Could you check a few things on this model? Use its own coordinates, in mm. A direction names the side the tool comes from. Give positions to 0.01 mm unless a question says otherwise; leave off trailing zeros. Loops run counter-clockwise (first coordinate to the right, second up) from the corner with the lowest first, then second, coordinate; pieces in that order, holes last. Notation, with made-up numbers: M 45,88 L 65,88 A29 ccw 65,124 Z; hole C 1.5,73.25 d9. An arc over 180 degrees is marked long. Answer in a Markdown table with one row per item. Add a question column.
1. Thinking about a two-plate mould opening in X: for faces 3 (the cylindrical face through (173.486, 211.797, -0.76)), 4 (the flat face through (128, 106, -1.5)), 5 (the cylindrical face through (247.34, 11.55, -0.76)), 6 (the cylindrical face through (4.51, 248.22, -0.76)), which applies, released by +X, released by -X, zero draft, split by the parting line, or undercut?
2. If we section it at A-A on x = 57.5: List the corners of the cut face in (y, z) for me.
3. I need wall thicknesses on line 1 along X through (y, z) = (257.5, -0.4); line 2 along Y through (x, z) = (19.5, -1.1); line 3 along X through (y, z) = (221.5, -1). Which ranges of each line are inside material? Lowest first, please. Write a range as from..to.
4. Which directions (+Z, -Z, +X, -X, +Y, -Y) give clear straight access to the entire face, cutting with the end or side of a thin tool? Please do faces 1 (the cylindrical face through (197.01, 265.15, -0.76)), 2 (the cylindrical face through (85.203, 211.486, -0.76)).
5. If we section it at B-B on z = -1.05: Count the separate pieces of the cut face and the enclosed holes in it, then the cut area to 3 significant figures.
```python
from build123d import *

# Parameters (mm, degrees)
CONVERT_SOLID1_START       = -1.5
CONVERT_SOLID1_OUTLINE_R   = 2.6
CONVERT_SOLID1_OUTLINE_R_2 = 1.65
CONVERT_SOLID1_OUTLINE_R_3 = 3.5
CONVERT_SOLID1_OUTLINE_R_4 = 10
CONVERT_SOLID1_DEPTH       = 1.5


# Read off the part's stored shape, not the designer's step: Convert-Solid1
with BuildPart() as part:
    # Convert-Solid1 outline → Convert-Solid1 (new body)
    with BuildSketch(Plane.XY.offset(CONVERT_SOLID1_START)):
        with BuildLine():
            ThreePointArc((204, 268), (196.928932188, 265.071067812), (194, 258))
            Line((194, 258), (194, 253))
            ThreePointArc((194, 253), (193.853553391, 252.646446609), (193.5, 252.5))
            Line((193.5, 252.5), (15, 252.5))
            ThreePointArc((15, 252.5), (4.393398282, 248.106601718), (0, 237.5))
            Line((0, 237.5), (0, 30.5))
            ThreePointArc((0, 30.5), (4.393398282, 19.893398282), (15, 15.5))
            Line((15, 15.5), (193.5, 15.5))
            ThreePointArc((193.5, 15.5), (193.853553391, 15.353553391), (194, 15))
            Line((194, 15), (194, 10))
            ThreePointArc((194, 10), (196.928932188, 2.928932188), (204, 0))
            Line((204, 0), (249, 0))
            ThreePointArc((249, 0), (256.071067812, 2.928932188), (259, 10))
            Line((259, 10), (259, 258))
            ThreePointArc((259, 258), (256.071067812, 265.071067812), (249, 268))
            Line((249, 268), (204, 268))
        make_face()
        with Locations((10.5, 50)):
            Circle(CONVERT_SOLID1_OUTLINE_R, mode=Mode.SUBTRACT)
        with Locations((19.5, 60.5)):
            Circle(CONVERT_SOLID1_OUTLINE_R, mode=Mode.SUBTRACT)
        with Locations((10.5, 71)):
            Circle(CONVERT_SOLID1_OUTLINE_R, mode=Mode.SUBTRACT)
        with Locations((82.529437252, 120.529437252)):
            Circle(CONVERT_SOLID1_OUTLINE_R_2, mode=Mode.SUBTRACT)
        with Locations((209, 10.5)):
            Circle(CONVERT_SOLID1_OUTLINE_R_3, mode=Mode.SUBTRACT)
        with Locations((218.380820142, 10.5)):
            Circle(CONVERT_SOLID1_OUTLINE_R_2, mode=Mode.SUBTRACT)
        with Locations((233.880820142, 10.5)):
            Circle(CONVERT_SOLID1_OUTLINE_R_2, mode=Mode.SUBTRACT)
        with Locations((244, 10.5)):
            Circle(CONVERT_SOLID1_OUTLINE_R_3, mode=Mode.SUBTRACT)
        with Locations((212.5, 46.5)):
            Circle(CONVERT_SOLID1_OUTLINE_R_2, mode=Mode.SUBTRACT)
        with Locations((226.5, 60.5)):
            Circle(CONVERT_SOLID1_OUTLINE_R_4, mode=Mode.SUBTRACT)
        with Locations((240.5, 46.5)):
            Circle(CONVERT_SOLID1_OUTLINE_R_2, mode=Mode.SUBTRACT)
        with Locations((129.5, 113.5)):
            Circle(CONVERT_SOLID1_OUTLINE_R_2, mode=Mode.SUBTRACT)
        with Locations((176.470562748, 120.529437252)):
            Circle(CONVERT_SOLID1_OUTLINE_R_2, mode=Mode.SUBTRACT)
        with Locations((212.5, 74.5)):
            Circle(CONVERT_SOLID1_OUTLINE_R_2, mode=Mode.SUBTRACT)
        with Locations((240.5, 74.5)):
            Circle(CONVERT_SOLID1_OUTLINE_R_2, mode=Mode.SUBTRACT)
        with Locations((10.5, 197)):
            Circle(CONVERT_SOLID1_OUTLINE_R, mode=Mode.SUBTRACT)
        with Locations((75.5, 167.5)):
            Circle(CONVERT_SOLID1_OUTLINE_R_2, mode=Mode.SUBTRACT)
        with Locations((19.5, 207.5)):
            Circle(CONVERT_SOLID1_OUTLINE_R, mode=Mode.SUBTRACT)
        with Locations((10.5, 218)):
            Circle(CONVERT_SOLID1_OUTLINE_R, mode=Mode.SUBTRACT)
        with Locations((82.529437252, 214.470562748)):
            Circle(CONVERT_SOLID1_OUTLINE_R_2, mode=Mode.SUBTRACT)
        with BuildLine():
            Line((179.5, 197.5), (179.5, 137.5))
            ThreePointArc((179.5, 137.5), (173.642135624, 123.357864376), (159.5, 117.5))
            Line((159.5, 117.5), (99.5, 117.5))
            ThreePointArc((99.5, 117.5), (85.357864376, 123.357864376), (79.5, 137.5))
            Line((79.5, 137.5), (79.5, 197.5))
            ThreePointArc((79.5, 197.5), (85.357864376, 211.642135624), (99.5, 217.5))
            Line((99.5, 217.5), (159.5, 217.5))
            ThreePointArc((159.5, 217.5), (173.642135624, 211.642135624), (179.5, 197.5))
        make_face(mode=Mode.SUBTRACT)
        with Locations((183.5, 167.5)):
            Circle(CONVERT_SOLID1_OUTLINE_R_2, mode=Mode.SUBTRACT)
        with Locations((212.5, 193.5)):
            Circle(CONVERT_SOLID1_OUTLINE_R_2, mode=Mode.SUBTRACT)
        with Locations((240.5, 193.5)):
            Circle(CONVERT_SOLID1_OUTLINE_R_2, mode=Mode.SUBTRACT)
        with Locations((129.5, 221.5)):
            Circle(CONVERT_SOLID1_OUTLINE_R_2, mode=Mode.SUBTRACT)
        with Locations((176.470562748, 214.470562748)):
            Circle(CONVERT_SOLID1_OUTLINE_R_2, mode=Mode.SUBTRACT)
        with Locations((226.5, 207.5)):
            Circle(CONVERT_SOLID1_OUTLINE_R_4, mode=Mode.SUBTRACT)
        with Locations((212.5, 221.5)):
            Circle(CONVERT_SOLID1_OUTLINE_R_2, mode=Mode.SUBTRACT)
        with Locations((240.5, 221.5)):
            Circle(CONVERT_SOLID1_OUTLINE_R_2, mode=Mode.SUBTRACT)
        with Locations((209, 257.5)):
            Circle(CONVERT_SOLID1_OUTLINE_R_3, mode=Mode.SUBTRACT)
        with Locations((218.75, 257.5)):
            Circle(CONVERT_SOLID1_OUTLINE_R_2, mode=Mode.SUBTRACT)
        with Locations((234.25, 257.5)):
            Circle(CONVERT_SOLID1_OUTLINE_R_2, mode=Mode.SUBTRACT)
        with Locations((244, 257.5)):
            Circle(CONVERT_SOLID1_OUTLINE_R_3, mode=Mode.SUBTRACT)
    extrude(amount=CONVERT_SOLID1_DEPTH)


solid = part.part
```
Results:
| question | item | result |
|---|---|---|
| 1 | face 3 | undercut |
| 1 | face 4 | zero draft |
| 1 | face 5 | undercut |
| 1 | face 6 | released by -X |
| 2 | outline | M 15.5,-1.5 L 252.5,-1.5 L 252.5,0 L 15.5,0 Z |
| 3 | line 1 | 194..205.5, 212.5..217.1, 220.4..232.6, 235.9..240.5, 247.5..259 |
| 3 | line 2 | 15.5..57.9, 63.1..204.9, 210.1..252.5 |
| 3 | line 3 | 0..127.85, 131.15..210.85, 214.15..238.85, 242.15..259 |
| 4 | face 1 | +Z, -Z, -X, +Y |
| 4 | face 2 | +Z, -Z |
| 5 | separate pieces | 1 |
| 5 | enclosed holes | 33 |
| 5 | area | 52,500 mm2 |
